Job drawing, mm, ordinate dimensions from the low corner. One solid piece. A direction names the side the tool comes from. Coordinates: 2 decimals unless noted, no trailing zeros. Loops run counter-clockwise (first coordinate to the right, second up) from the corner with the lowest first, then second, coordinate; pieces in that order, holes last. Notation, with made-up numbers: (-7, 17.5) - (7, 17.5) arc R31 ccw to (7, 51.5) - close; hole circle Ø11 at (88.5, 18.25). An arc over 180 degrees is marked (long way). Use a Markdown table: item, result. Add a question column.
1) Drop flat-ended pins along their axis: P1, Ø10, axis at x = 15, z = 14.5, coming from the +Y side; P2, Ø8, axis at x = 7, y = 15, coming from the +Z side; P3, Ø3, axis at x = 12, y = 4.5, coming from the +Z side. Give the stop position or say it passes through.
2) Band-saw the part on D-D (z = 3.25). Give the cut face in (x, y).
3) Band-saw the part on A-A (z = 19). Give the cut face in (x, y), plus the area to 3 significant figures.
4) Band-saw the part on C-C (x = 12.75). Give the cut face in (y, z) (3 decimals), plus the area to 3 significant figures.
5) Pull direction X, two halves, no side cores. Call the marked faces 4, 5 and 6: +X half, -X half, draft (parallel to the pull), parting line (faces both ways), or undercut.
6) Band-saw the part on B-B (y = 1.75). Give the cut face in (x, z).
7) Tool access for the marked faces 1, 2 and 3: list every direction of +Z, -Z, +X, -X, +Y, -Y with a clear straight run to the whole face (end or side of a thin tool).
8) Probe probe 1 along Z at (x, y) = (15.75, 14.5); probe 2 along X at (y, z) = (9.5, 23). List the from-to ranges inside material, lowest first. Write a range as [from, to].
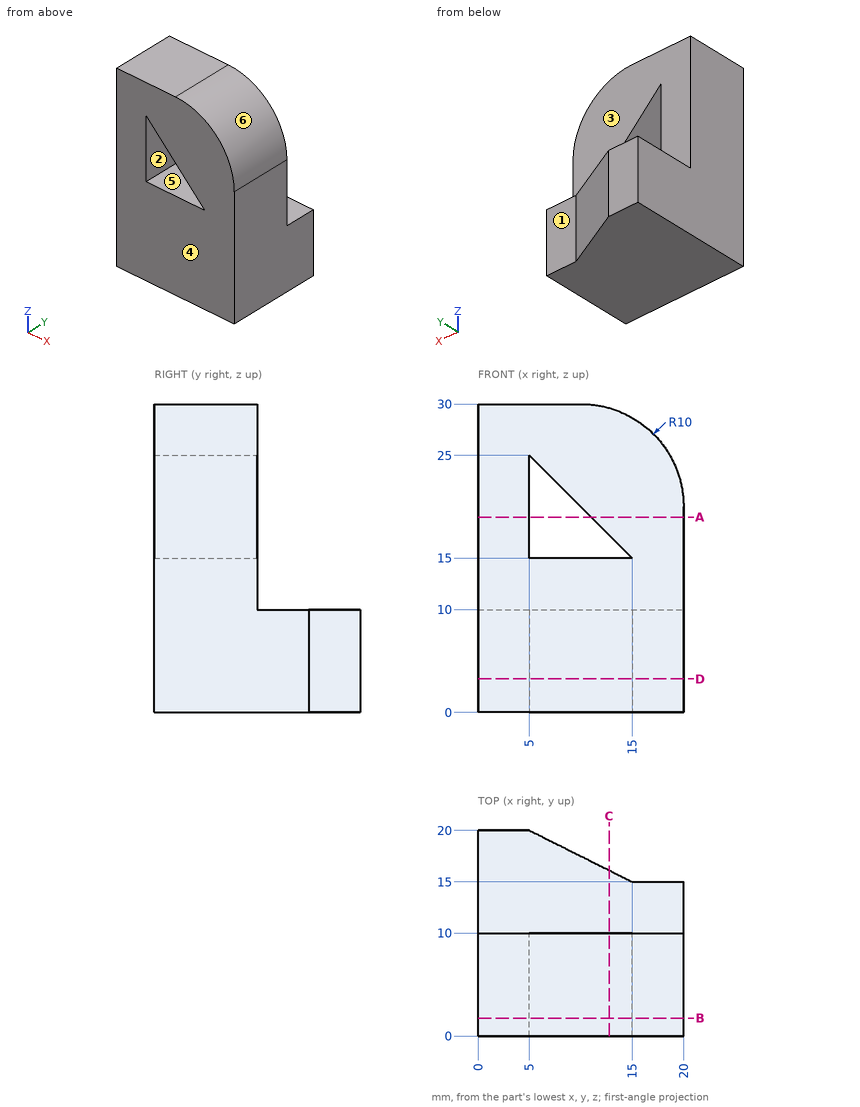
Answer block:
| question | item | result |
|---|---|---|
| 1 | P1 | y = 16.09 |
| 1 | P2 | z = 10 |
| 1 | P3 | z = 29.99 |
| 2 | outline | (0, 0) - (20, 0) - (20, 15) - (15, 15) - (5, 20) - (0, 20) - close |
| 3 | outline | (0, 0) - (5, 0) - (5, 10) - (0, 10) - close; (11, 0) - (20, 0) - (20, 10) - (11, 10) - close |
| 3 | area | 140 mm2 |
| 4 | outline | (0, 0) - (16.125, 0) - (16.125, 10) - (10, 10) - (10, 15) - (0, 15) - close; (0, 17.25) - (10, 17.25) - (10, 29.614) - (0, 29.614) - close |
| 4 | area | 335 mm2 |
| 5 | face 4 | draft |
| 5 | face 5 | undercut |
| 5 | face 6 | +X half |
| 6 | outline | (0, 0) - (20, 0) - (20, 20) arc R10 ccw to (10, 30) - (0, 30) - close; hole (5, 15) - (15, 15) - (5, 25) - close |
| 7 | face 1 | +Z, -Z, +X, +Y |
| 7 | face 2 | +Y, -Y |
| 7 | face 3 | +Z, +X, -X, +Y |
| 8 | probe 1 | [0, 10] |
| 8 | probe 2 | [0, 5], [7, 19.54] |
